from build123d import *

# Parameters (mm, degrees)
EXTRUDE_1_DEPTH     = 5
SKETCH_3_R          = 5.55
CUT_EXTRUDE_1_DEPTH = 5
FILLET_1_R          = 5
SKETCH_4_R          = 6.5
CUT_EXTRUDE_2_DEPTH = 0.6


with BuildPart() as part:
    # 草图1 → 凸台-拉伸1 (new body)
    with BuildSketch(Plane.XY):
        with BuildLine():
            ThreePointArc((-7.931682852, -1.043267527), (7.134318966, -3.619598443), (-3.842383801, 7.016843074))
            ThreePointArc((-3.842383801, 7.016843074), (-19, 10), (-34.157616199, 7.016843074))
            ThreePointArc((-34.157616199, 7.016843074), (-45.134318966, -3.619598443), (-30.068317148, -1.043267527))
            ThreePointArc((-30.068317148, -1.043267527), (-19, 1), (-7.931682852, -1.043267527))
        make_face()
    extrude(amount=-EXTRUDE_1_DEPTH)

    # 草图3 → 切除-拉伸1 (cut)
    with BuildSketch(Plane(origin=(0, 0, -5), x_dir=(-1, 0, 0), z_dir=(0, 0, -1))):
        Circle(SKETCH_3_R)
        with Locations((38, 0)):
            Circle(SKETCH_3_R)
    extrude(amount=-CUT_EXTRUDE_1_DEPTH, mode=Mode.SUBTRACT)

    # 圆角1
    fillet_1_edges = [part.edges().sort_by_distance(p)[0] for p in [
        (-30.068317148, -1.043267527, -2.5),
        (-34.157616199, 7.016843074, -2.5),
        (-3.842383801, 7.016843074, -2.5),
        (-7.931682852, -1.043267527, -2.5),
    ]]
    fillet(fillet_1_edges, radius=FILLET_1_R)

    # 草图4 → 切除-拉伸2 (cut)
    with BuildSketch(Plane.XY):
        with Locations((-38, 0)):
            Circle(SKETCH_4_R)
    extrude(amount=-CUT_EXTRUDE_2_DEPTH, mode=Mode.SUBTRACT)


solid = part.part
CAD build for the part. Positions are in the model's coordinates, mm. A direction names the side the tool comes from. Coordinates: 2 decimals unless noted, no trailing zeros. Write each loop counter-clockwise with the first axis right and the second up, starting at its lowest first coordinate (ties: lowest second). Pieces come first, ordered by that corner, then holes. Notation, with made-up numbers: (48.25, 88.25) - (80.25, 88.25) arc R20 cw to (80.25, 114.25) - close; hole circle Ø8 at (55.25, 12.5). An arc over 180 degrees is marked (long way). Use a Markdown table: item, result. Add a question column.
Item 1: Band-saw the part on B-B, the plane y = 0.5. Give the cut face in (x, z), and give its area (3 significant figures).
Item 2: Drill centre lines: L1, parallel to Y at x = -38, z = -1.9; L2, parallel to X at y = -5, z = -1.3 (3 decimals); L3, parallel to X at y = 3.75, z = -1.55. Where is each one in solid material? Low to high. Write a range as from..to.
Item 3: 3-axis set-ups, long thin cutter, end or side, ignore diameter. For faces 3 (the face through (-19, 3, 0)), 4 (the face through (-44.494, 0.286, -0.296)): which of +Z, -Z, +X, -X, +Y, -Y reach the whole face in a straight line?
Item 4: Flat gauge pins, fed straight in: pin 1 (1.5 mm diameter, centred on y = 3, z = -3.5, fed in from -X); pin 2 (6.5 mm diameter, centred on x = -38, y = 0, fed in from -Z). Where does each tip first touch, or does it go through?
Item 5: Band-saw the part on D-D, the plane z = -2.3. Give the number of separate pieces and of enclosed holes in the cut face, and give its area (3 significant figures).
Item 6: Mould opens along X. For faces 1 (the face through (-33, 3, -0.6)), 2 (the face through (-19, 3, -5)) say: pulls with the +X half, pulls with the -X half, needs draft (parallel to the pull), parting line crosses it, or undercut.
Item 7: Band-saw the part on A-A, the plane x = -38. Give the cut face in (y, z), and give its area (3 significant figures).
Item 8: Band-saw the part on C-C, the plane x = 0. Give the cut face in (y, z), and give its area (3 significant figures).
Numbers:
| question | item | result |
|---|---|---|
| 1 | outline | (-45.98, -5) - (-43.53, -5) - (-43.53, -0.6) - (-44.48, -0.6) - (-44.48, 0) - (-45.98, 0) - close; (-32.47, -5) - (-24.55, -5) - (-24.55, 0) - (-31.52, 0) - (-31.52, -0.6) - (-32.47, -0.6) - close; (-13.45, -5) - (-5.53, -5) - (-5.53, 0) - (-13.45, 0) - close; (5.53, -5) - (7.98, -5) - (7.98, 0) - (5.53, 0) - close |
| 1 | area | 103 mm2 |
| 2 | L1 | -8..-5.55, 5.55..8 |
| 2 | L2 | -44.245..-40.409, -35.591..-31.755, -6.245..-2.409, 2.409..6.245 |
| 2 | L3 | -45.07..-42.09, -33.91..-4.09, 4.09..7.07 |
| 3 | face 3 | +Z, +X, -X, +Y, -Y |
| 3 | face 4 | +Z |
| 4 | pin 1 | x = -45.68 |
| 4 | pin 2 | through |
| 5 | separate pieces | 1 |
| 5 | enclosed holes | 2 |
| 5 | area | 436 mm2 |
| 6 | face 1 | undercut |
| 6 | face 2 | needs draft |
| 7 | outline | (-8, -5) - (-5.55, -5) - (-5.55, -0.6) - (-6.5, -0.6) - (-6.5, 0) - (-8, 0) - close; (5.55, -5) - (8, -5) - (8, 0) - (6.5, 0) - (6.5, -0.6) - (5.55, -0.6) - close |
| 7 | area | 23.4 mm2 |
| 8 | outline | (-8, -5) - (-5.55, -5) - (-5.55, 0) - (-8, 0) - close; (5.55, -5) - (8, -5) - (8, 0) - (5.55, 0) - close |
| 8 | area | 24.5 mm2 |
